from build123d import *

# Parameters (mm, degrees)
SKETCH1_R           = 5.5
SKETCH1_R_2         = 2.5
BOSS_EXTRUDE1_DEPTH = 8
BOSS_EXTRUDE2_START = -8
BOSS_EXTRUDE2_DEPTH = 8
SKETCH3_R           = 2
CUT_EXTRUDE1_DEPTH  = 8


with BuildPart() as part:
    # Sketch1 → Boss-Extrude1 (new body)
    with BuildSketch(Plane(origin=(0, 0, 0), x_dir=(1, 0, 0), z_dir=(0, 1, 0))):
        with Locations(Location((0, 0, 0), (0, 0, 270))):
            Circle(SKETCH1_R)
        with Locations(Location((0, 0, 0), (0, 0, 270))):
            Circle(SKETCH1_R_2, mode=Mode.SUBTRACT)
    extrude(amount=BOSS_EXTRUDE1_DEPTH)

    # Sketch2 → Boss-Extrude2 (add)
    with BuildSketch(Plane(origin=(0, 8, 0), x_dir=(1, 0, 0), z_dir=(0, 1, 0)).offset(BOSS_EXTRUDE2_START)):
        with BuildLine():
            Line((15, -4.5), (6.662278045, -4.5))
            Line((6.662278045, -4.5), (3.16227766, -4.5))
            ThreePointArc((3.16227766, -4.5), (1.658312395, -5.244044241), (0, -5.5))
            Line((0, -5.5), (0, -7.5))
            Line((0, -7.5), (15, -7.5))
            Line((15, -7.5), (15, -4.5))
        make_face()
        with BuildLine():
            Line((6.662278045, -4.5), (5.4823084, 0.440788615))
            ThreePointArc((5.4823084, 0.440788615), (5.49557532, 0.220571755), (5.5, 0))
            ThreePointArc((5.5, 0), (4.880703184, -2.535495304), (3.16227766, -4.5))
            Line((3.16227766, -4.5), (6.662278045, -4.5))
        make_face()
        with BuildLine():
            ThreePointArc((-3.16227766, -4.5), (-4.978460111, -2.337720027), (-5.4823084, 0.440788615))
            Line((-5.4823084, 0.440788615), (-6.662278045, -4.5))
            Line((-6.662278045, -4.5), (-3.16227766, -4.5))
        make_face()
        with BuildLine():
            Line((-3.16227766, -4.5), (-6.662278045, -4.5))
            Line((-6.662278045, -4.5), (-15, -4.5))
            Line((-15, -4.5), (-15, -7.5))
            Line((-15, -7.5), (0, -7.5))
            Line((0, -7.5), (0, -5.5))
            ThreePointArc((0, -5.5), (-1.658312395, -5.244044241), (-3.16227766, -4.5))
        make_face()
    extrude(amount=BOSS_EXTRUDE2_DEPTH)

    # Sketch3 → Cut-Extrude1 (cut)
    with BuildSketch(Plane(origin=(0, 0, 4.5), x_dir=(-1, 0, 0), z_dir=(0, 0, -1))):
        with BuildLine():
            ThreePointArc((-8.831139022, 4), (-10.831139022, 6), (-12.831139022, 4))
            Line((-12.831139022, 4), (-8.831139022, 4))
        make_face()
        with BuildLine():
            Line((-8.831139022, 4), (-12.831139022, 4))
            ThreePointArc((-12.831139022, 4), (-10.831139022, 2), (-8.831139022, 4))
        make_face()
        with Locations((10.831139022, 4)):
            Circle(SKETCH3_R)
    extrude(amount=-CUT_EXTRUDE1_DEPTH, mode=Mode.SUBTRACT)


solid = part.part
Model file for the job. Use its own axes, mm. A direction names the side the tool comes from. Give positions to 0.01 mm unless a question says otherwise; leave off trailing zeros. Loops run counter-clockwise (first coordinate to the right, second up) from the corner with the lowest first, then second, coordinate; pieces in that order, holes last. Notation, with made-up numbers: (45, 13) -> (70, 13) arc R17 cw to (70, 43) -> close; hole circle Ø2 at (3, 58). An arc over 180 degrees is marked (long way). Use a Markdown table: item, result. Add a question column.
(1) Slice it at D-D on z = 0. List the corners of the cut face in (x, y).
(2) Slice it at A-A on y = 4. List the corners of the cut face in (x, z), and give its area (3 significant figures).
(3) Drop flat-ended pins along their axis: pin 1 Ø3 at (x, z) = (7.5, 3.5) entering from -Y; pin 2 Ø3 at (x, y) = (10.83, 4) entering from -Z; pin 3 Ø4 at (y, z) = (1.5, 0.5) entering from -X. Give the stop position or say it passes through.
(4) Wall check: line 1 along X through (y, z) = (2.25, -0.25); line 2 along Z through (x, y) = (-10.25, 6.5); line 3 along X through (y, z) = (0.5, -1.5). Give the ranges that are in metal, low to high.
(5) Mould opens along Z. For faces 1 (the flat face through (0, 8, 4)), 2 (the flat face through (6.08, 3.94, 2.06)), 3 (the cylindrical face through (-2.44, 3.94, -0.54)) say: +Z half, -Z half, draft (parallel to the pull), parting line (faces both ways), or undercut.
(6) Slice it at C-C on y = 6.5. List the corners of the cut face in (x, z), and give its area (3 significant figures).
(7) Slice it at B-B on x = 0. List the corners of the cut face in (y, z), and give its area (3 significant figures).
(8) Tool access for faces 4 (the cylindrical face through (8.833, 3.912, 5.979)), 5 (the flat face through (12, 2, 4.5)), 6 (the flat face through (-10, 2, 4.5)): list every direction of +Z, -Z, +X, -X, +Y, -Y with a clear straight run to the whole face (end or side of a thin tool).
Filled sheet:
| question | item | result |
|---|---|---|
| 1 | outline | (-5.59, 0) -> (-2.5, 0) -> (-2.5, 8) -> (-5.59, 8) -> close; (2.5, 0) -> (5.59, 0) -> (5.59, 8) -> (2.5, 8) -> close |
| 2 | outline | (-15, 4.5) -> (-12.83, 4.5) -> (-12.83, 7.5) -> (-15, 7.5) -> close; (-8.83, 4.5) -> (-6.66, 4.5) -> (-5.48, -0.44) arc R5.5 ccw to (5.48, -0.44) -> (6.66, 4.5) -> (8.83, 4.5) -> (8.83, 7.5) -> (-8.83, 7.5) -> close; (12.83, 4.5) -> (15, 4.5) -> (15, 7.5) -> (12.83, 7.5) -> close; hole circle Ø5 at (0, 0) |
| 2 | area | 149 mm2 |
| 3 | pin 1 | y = 0 |
| 3 | pin 2 | through |
| 3 | pin 3 | x = -6.18 |
| 4 | line 1 | -5.53 to -2.49, 2.49 to 5.53 |
| 4 | line 2 | 4.5 to 7.5 |
| 4 | line 3 | -5.29 to -2, 2 to 5.29 |
| 5 | face 1 | draft |
| 5 | face 2 | -Z half |
| 5 | face 3 | undercut |
| 6 | outline | (-15, 4.5) -> (-6.66, 4.5) -> (-5.48, -0.44) arc R5.5 ccw to (5.48, -0.44) -> (6.66, 4.5) -> (15, 4.5) -> (15, 7.5) -> (-15, 7.5) -> close; hole circle Ø5 at (0, 0) |
| 6 | area | 173 mm2 |
| 7 | outline | (0, -5.5) -> (8, -5.5) -> (8, -2.5) -> (0, -2.5) -> close; (0, 2.5) -> (8, 2.5) -> (8, 7.5) -> (0, 7.5) -> close |
| 7 | area | 64.0 mm2 |
| 8 | face 4 | +Z, -Z |
| 8 | face 5 | -Z, +X, +Y, -Y |
| 8 | face 6 | -Z, -X, +Y, -Y |
